Autodesk Inventor part; units mm, degrees
ref_plane "YZ Plane" through (0, 0, 0) normal (1, 0, 0) x (0, 1, 0)
ref_plane "XZ Plane" through (0, 0, 0) normal (0, 1, 0) x (-1, 0, 0)
ref_plane "XY Plane" through (0, 0, 0) normal (0, 0, 1) x (1, 0, 0)
sketch "Sketch1" plane through (0, 0, 0) normal (0, 1, 0) x (-1, 0, 0)
  circle A0 centre (0, 0) radius 80
  dimension "d0" = 160
extrude "Extrusion1" add sketch "Sketch1" along normal blind 10
sketch "Sketch2" plane through (0, 10, 0) normal (0, 1, 0) x (1, 0, 0)
  circle A0 centre (0, 0) radius 17.5
  dimension "d5" = 35
extrude "Extrusion2" cut sketch "Sketch2" against normal blind 10
sketch "Sketch3" plane through (0, 10, 0) normal (0, 1, 0) x (1, 0, 0)
  circle A0 centre (0, 0) radius 40
  dimension "d8" = 80
extrude "Extrusion3" cut sketch "Sketch3" against normal blind 5
fillet "Fillet2" radius 5 1 edges at (-17.5, 5, 0)
properties part number "faceplate" material "Stainless Steel"
Geometry check sheet. Reference: the model listing, model coordinates, mm. Coordinates: 2 decimals unless noted, no trailing zeros. Order: outer loops, then holes, each group sorted by start corner. A loop starts at its lowest first (then second) coordinate and runs counter-clockwise, first axis right, second up. Notation, with made-up numbers: (-19, 40) - (-14, 40) arc R16 cw to (-14, 56) - close; hole circle Ø7 at (16, -39). An arc over 180 degrees is marked (long way). Use one line per item in the form item = value.
1. Section check C-C (y = 8). Record the boundary of the cut face in (x, z), then the cut area to 3 significant figures.
Here are the results:
outline = circle Ø160 at (0, 0); hole circle Ø80 at (0, 0)
area = 15,100 mm²
2. Draft check along Z on faces 1 (the face through (-17, 10, 37)), 2 (the face through (-8.67, 7.54, 39.05)), 3 (the face through (17.34, 4.93, 78.1)), 4 (the face through (17, 5, 17)). Enter one of: pulls with the +Z half, pulls with the -Z half, needs draft (parallel to the pull), parting line crosses it, or undercut.
Here are the results:
face_1 = needs draft
face_2 = undercut
face_3 = parting line crosses it
face_4 = undercut
3. Scan lines: line 1 (Z direction, x = 0, y = 0.05); line 2 (Z direction, x = 0, y = 6.4); line 3 (Y direction, x = 7.5, z = 34). Record each from-to range of solid material in increasing order.
Here are the results:
line_1 = -80 to -17.5, 17.5 to 80
line_2 = -80 to -40, 40 to 80
line_3 = 0 to 5
4. Section check D-D (x = -64). Record the boundary of the cut face in (y, z), then the cut area to 3 significant figures.
Here are the results:
outline = (0, -48) - (10, -48) - (10, 48) - (0, 48) - close
area = 960 mm²
5. Gauge pin test, flat ends, axial feed: pin 1 (3 mm diameter, centred on x = 14, y = 7.5, fed in from +Z); pin 2 (1 mm diameter, centred on x = 14.5, y = 8.5, fed in from +Z); pin 3 (6 mm diameter, centred on x = 43, y = 1.5, fed in from +Z). Record the tip position at first contact, or that the pin passes through.
Here are the results:
pin_1 = 79.02
pin_2 = 78.77
pin_3 = 69.28
